Part print with two shaded views. Sizes in mm from the minimum x, y, z corner. Round coordinates to 2 decimals unless told otherwise and drop trailing zeros. Write each loop counter-clockwise with the first axis right and the second up, starting at its lowest first coordinate (ties: lowest second). Pieces come first, ordered by that corner, then holes. Notation, with made-up numbers: (88.5, 30) - (122.5, 30) arc R31 cw to (122.5, 54) - close; hole circle Ø6 at (20, 35). An arc over 180 degrees is marked (long way). Use one line per item in the form item = value. Start each with the question number.
Item 1: Band-saw the part on A-A, the plane y = 48. List the corners of the cut face in (x, z) (3 decimals), and give its area (3 significant figures).
Item 2: Band-saw the part on B-B, the plane x = 87. List the corners of the cut face in (y, z), and give its area (3 significant figures).
Item 3: Drill centre lines: L1, parallel to X at y = 22, z = 5 (3 decimals); L2, parallel to X at y = 37, z = 5 (3 decimals); L3, parallel to X at y = 56, z = 3. Where is each one in solid material? Low to high.
Item 4: Pin check, flat tips, straight feed: pin 1 (5 mm diameter, centred on y = 44, z = 3, fed in from -X); pin 2 (5 mm diameter, centred on x = 74.5, z = 5.5, fed in from +Y); pin 3 (1.8 mm diameter, centred on x = 120, z = 5, fed in from -Y). Stop position of each tip, or through.
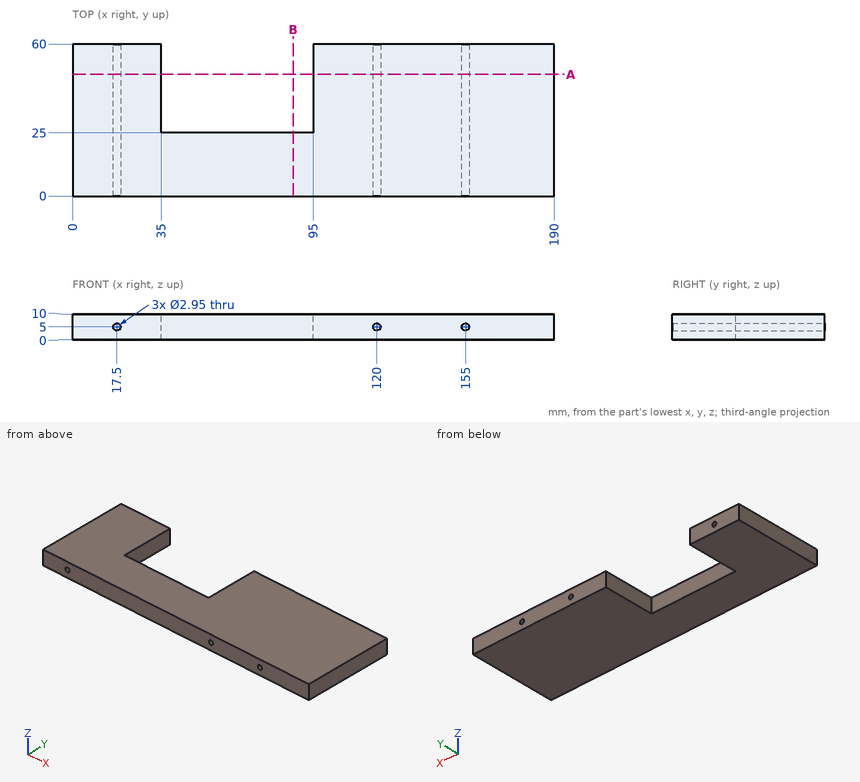
Determined:
q1.outline = (0, 0) - (35, 0) - (35, 10) - (0, 10) - close; (95, 0) - (190, 0) - (190, 10) - (95, 10) - close; hole circle Ø2.95 at (17.5, 5); hole circle Ø2.95 at (120, 5); hole circle Ø2.95 at (155, 5)
q1.area = 1,280 mm²
q2.outline = (0, 0) - (25, 0) - (25, 10) - (0, 10) - close
q2.area = 250 mm²
q3.L1 = 0 to 16.025, 18.975 to 118.525, 121.475 to 153.525, 156.475 to 190
q3.L2 = 0 to 16.025, 18.975 to 35, 95 to 118.525, 121.475 to 153.525, 156.475 to 190
q3.L3 = 0 to 35, 95 to 190
q4.pin_1 = 0
q4.pin_2 = 25
q4.pin_3 = through
